Geometry check sheet. Reference: the model listing, model coordinates, mm. A direction names the side the tool comes from. Coordinates: 2 decimals unless noted, no trailing zeros. Write each loop counter-clockwise with the first axis right and the second up, starting at its lowest first coordinate (ties: lowest second). Pieces come first, ordered by that corner, then holes. Notation, with made-up numbers: M 75.25,57 L 95.25,57 A22 ccw 95.25,86 Z; hole C 4.5,30 d9. An arc over 180 degrees is marked long. Answer as a JSON object with one key per item and string values. Group by question number.
```python
from build123d import *

# Parameters (mm, degrees)
SKETCH1_R           = 6
SKETCH1_R_2         = 1.5
BOSS_EXTRUDE1_DEPTH = 3.175


with BuildPart() as part:
    # Sketch1 → Boss-Extrude1 (new body)
    with BuildSketch(Plane.XY):
        Polygon((18.5, 0), (37, 0), (37, 37), (18.5, 37), (18.5, 43.35), (0, 43.35), (0, 37), (0, 0), align=None)
        with Locations((18.39023312, 12.089873912)):
            Circle(SKETCH1_R, mode=Mode.SUBTRACT)
        with Locations((2.89023312, 19.089873912)):
            Circle(SKETCH1_R_2, mode=Mode.SUBTRACT)
        with Locations((10.64023312, 5.666480153)):
            Circle(SKETCH1_R_2, mode=Mode.SUBTRACT)
        with Locations((26.14023312, 5.666480153)):
            Circle(SKETCH1_R_2, mode=Mode.SUBTRACT)
        with Locations((33.89023312, 19.089873912)):
            Circle(SKETCH1_R_2, mode=Mode.SUBTRACT)
        with Locations((26.14023312, 32.513267671)):
            Circle(SKETCH1_R_2, mode=Mode.SUBTRACT)
        with Locations((10.64023312, 32.513267671)):
            Circle(SKETCH1_R_2, mode=Mode.SUBTRACT)
    extrude(amount=BOSS_EXTRUDE1_DEPTH)


solid = part.part
```
1) Material ranges on probe 1 along Y at (x, z) = (10.5, 0.6); probe 2 along Y at (x, z) = (11, 0.3); probe 3 along Y at (x, z) = (30, 1.9), recorded low to high. Write a range as [from, to].
2) Section check A-A (y = 13.5). Record the cut outline in (x, z) (3 decimals), then the cut area to 3 significant figures.
3) Section check B-B (x = 23). Record the cut outline in (y, z) (3 decimals).
4) Set-up check for faces 5 (the flat face through (28, 37, 2)), 6 (the flat face through (18, 22, 3.175)): record each of +Z, -Z, +X, -X, +Y, -Y from which the full face is reachable in a straight line by a thin tool's end or side.
5) Draft check along X on faces 1 (the cylindrical face through (23.93, 9.79, 1.57)), 2 (the flat face through (0, 22, 2)), 3 (the flat face through (18, 0, 2)), 4 (the flat face through (18.5, 40, 2)). Enter one of: +X half, -X half, draft (parallel to the pull), parting line (faces both ways), or undercut.
6) Section check D-D (y = 38). Record the cut outline in (x, z) (3 decimals).
7) Section check C-C (z = 1.7). Record the cut outline in (x, y).
Entries:
{
 "1": {"probe 1": "[0, 4.17], [7.16, 31.02], [34.01, 43.35]", "probe 2": "[0, 4.21], [7.12, 31.06], [33.97, 43.35]", "probe 3": "[0, 37]"},
 "2": {"outline": "M 0,0 L 12.558,0 L 12.558,3.175 L 0,3.175 Z; M 24.222,0 L 37,0 L 37,3.175 L 24.222,3.175 Z", "area": "80.4 mm^2"},
 "3": {"outline": "M 0,0 L 8.249,0 L 8.249,3.175 L 0,3.175 Z; M 15.93,0 L 37,0 L 37,3.175 L 15.93,3.175 Z"},
 "4": {"face 5": "+Z, -Z, +X, +Y", "face 6": "+Z, +X, -X, +Y, -Y"},
 "5": {"face 1": "undercut", "face 2": "-X half", "face 3": "draft", "face 4": "+X half"},
 "6": {"outline": "M 0,0 L 18.5,0 L 18.5,3.175 L 0,3.175 Z"},
 "7": {"outline": "M 0,0 L 37,0 L 37,37 L 18.5,37 L 18.5,43.35 L 0,43.35 Z; hole C 2.89,19.09 d3; hole C 10.64,5.67 d3; hole C 10.64,32.51 d3; hole C 18.39,12.09 d12; hole C 26.14,5.67 d3; hole C 26.14,32.51 d3; hole C 33.89,19.09 d3"}
}
